```python
from build123d import *

# Parameters (mm, degrees)
SKETCH_2_R          = 6.9
EXTRUDE_1_DEPTH     = 1.6
SKETCH_4_R          = 6
EXTRUDE_2_DEPTH     = 10
SKETCH_7_R          = 4.5
SKETCH_7_R_2        = 3.5
CUT_EXTRUDE_1_DEPTH = 0.5
CUT_EXTRUDE_2_DEPTH = 0.2
CHAMFER_1_SIZE      = 0.1
FILLET_1_R          = 0.2


# Read off the part's stored shape, not the designer's step: M12 机械螺纹 螺柱1
with BuildPart() as part:
    # 草图2 → 凸台-拉伸1 (new body)
    with BuildSketch(Plane.XY):
        Circle(SKETCH_2_R)
    extrude(amount=EXTRUDE_1_DEPTH)

    # 草图3 → 切除-旋转1 (revolve, cut)
    with BuildSketch(Plane(origin=(0, 0, 0), x_dir=(1, 0, 0), z_dir=(0, 1, 0))):
        Polygon((-6.9, -1.1), (-5, 0), (-6.9, 0), align=None)
    revolve(axis=Axis((0, 0, -2.565533084), (0, 0, 1)), mode=Mode.SUBTRACT)

    # 草图4 → 凸台-拉伸2 (add)
    with BuildSketch(Plane.XY.offset(1.6)):
        Circle(SKETCH_4_R)
    extrude(amount=EXTRUDE_2_DEPTH)

    # M12 机械螺纹 螺柱1 outline → M12 机械螺纹 螺柱1 (revolve, cut)
    with BuildSketch(Plane.XZ):
        Polygon((6, 11.6), (5.053, 11.6), (6, 10.653), align=None)
    revolve(axis=Axis((0, 0, 0), (0, 0, 1)), mode=Mode.SUBTRACT)

    # 草图7 → 切除-拉伸1 (cut)
    with BuildSketch(Plane(origin=(0, 0, 0), x_dir=(-1, 0, 0), z_dir=(0, 0, -1))):
        Circle(SKETCH_7_R)
        Circle(SKETCH_7_R_2, mode=Mode.SUBTRACT)
    extrude(amount=-CUT_EXTRUDE_1_DEPTH, mode=Mode.SUBTRACT)

    # 草图8 → 切除-拉伸2 (cut)
    with BuildSketch(Plane(origin=(0, 0, 0), x_dir=(-1, 0, 0), z_dir=(0, 0, -1))):
        with BuildLine():
            Line((1.320582444, 1.833045199), (1.379254836, 1.91448589))
            ThreePointArc((1.379254836, 1.91448589), (1.517822019, 1.996168929), (1.671723162, 1.949399054))
            ThreePointArc((1.671723162, 1.949399054), (0, -2.568037189), (-1.671723162, 1.949399054))
            ThreePointArc((-1.671723162, 1.949399054), (-1.517822019, 1.996168929), (-1.379254836, 1.91448589))
            Line((-1.379254836, 1.91448589), (-1.320582444, 1.833045199))
            ThreePointArc((-1.320582444, 1.833045199), (-1.284222156, 1.69280287), (-1.352094962, 1.564805747))
            ThreePointArc((-1.352094962, 1.564805747), (0, -2.068037189), (1.352094962, 1.564805747))
            ThreePointArc((1.352094962, 1.564805747), (1.284222156, 1.69280287), (1.320582444, 1.833045199))
        make_face()
        with BuildLine():
            Line((-0.050187239, 1.280793561), (0.050187239, 1.280793561))
            ThreePointArc((0.050187239, 1.280793561), (0.191608596, 1.339372204), (0.250187239, 1.480793561))
            Line((0.250187239, 1.480793561), (0.250187239, 2.558804723))
            ThreePointArc((0.250187239, 2.558804723), (0.191608596, 2.70022608), (0.050187239, 2.758804723))
            Line((0.050187239, 2.758804723), (-0.050187239, 2.758804723))
            ThreePointArc((-0.050187239, 2.758804723), (-0.191608596, 2.70022608), (-0.250187239, 2.558804723))
            Line((-0.250187239, 2.558804723), (-0.250187239, 1.480793561))
            ThreePointArc((-0.250187239, 1.480793561), (-0.191608596, 1.339372204), (-0.050187239, 1.280793561))
        make_face()
    extrude(amount=-CUT_EXTRUDE_2_DEPTH, mode=Mode.SUBTRACT)

    # 倒角1
    chamfer_1_edges = [part.edges().sort_by_distance(p)[0] for p in [
        (4.5, 0, 0),
        (3.5, 0, 0),
    ]]
    chamfer(chamfer_1_edges, length=CHAMFER_1_SIZE)

    # 圆角1
    fillet_1_edges = [part.edges().sort_by_distance(p)[0] for p in [
        (-6.9, 0, 1.6),
        (0, 6.9, 1.1),
    ]]
    fillet(fillet_1_edges, radius=FILLET_1_R)


solid = part.part
```
Could you check a few things on this model? Use its own coordinates, in mm. A direction names the side the tool comes from. Coordinates: 2 decimals unless noted, no trailing zeros. Write each loop counter-clockwise with the first axis right and the second up, starting at its lowest first coordinate (ties: lowest second). Pieces come first, ordered by that corner, then holes. Notation, with made-up numbers: (-34, 42) -> (-14, 42) arc R22 ccw to (-14, 56) -> close; hole circle Ø10 at (-19, 44.5). An arc over 180 degrees is marked (long way). Return JSON: item names as keys, results as strings.
(1) I'm going to push flat-ended pins straight in: pin 1 (2 mm diameter, centred on x = -3, z = 5.5, fed in from +Y); pin 2 (1 mm diameter, centred on y = -3, z = 4.5, fed in from +X); pin 3 (3 mm diameter, centred on y = -5, z = 2.5, fed in from +X). Where does each tip first touch, or does it pass through?
Numbers:
{"pin 1": "stops at y = 5.66", "pin 2": "stops at x = 5.45", "pin 3": "stops at x = 5.67"}
(2) I need wall thicknesses on L1, parallel to Y at x = 0, z = 0.25; L2, parallel to Y at x = 0, z = 0.3; L3, parallel to Z at x = -2, y = 1. Which ranges of each line are inside material? Lowest first, please.
Numbers:
{"L1": "y = -5.43 to -4.5, -3.5 to 3.5, 4.5 to 5.43", "L2": "y = -5.52 to -4.5, -3.5 to 3.5, 4.5 to 5.52", "L3": "z = 0.2 to 11.6"}
(3) Imagine slicing it at A-A, the plane z = 4. Please give me the cut outline in (x, y).
Numbers:
{"outline": "circle Ø12 at (0, 0)"}
(4) We'd pull the mould along Y, two halves only. Please class faces 1 (the cylindrical face through (0.59, 4.46, 0.3)), 2 (the flat face through (0, 0, 0)), 3 (the cylindrical face through (-6, 0, 6)): +Y half, -Y half, draft (parallel to the pull), parting line (faces both ways), or undercut.
Numbers:
{"face 1": "undercut", "face 2": "draft", "face 3": "parting line"}
(5) Which directions (+Z, -Z, +X, -X, +Y, -Y) give clear straight access to the entire face, cutting with the end or side of a thin tool? Please do faces 4 (the flat face through (0, 0, 11.6)), 5 (the cylindrical face through (-3.233, -1.341, 0.297)), 6 (the flat face through (-2, -6, 1.6)).
Numbers:
{"face 4": "+Z, +X, -X, +Y, -Y", "face 5": "-Z", "face 6": "+Z"}
